Here's how the part is built. I have some questions about the finished solid (model axes, mm). A direction names the side the tool comes from. Round coordinates to 2 decimals unless told otherwise and drop trailing zeros. Loops run counter-clockwise (first coordinate to the right, second up) from the corner with the lowest first, then second, coordinate; pieces in that order, holes last. Notation, with made-up numbers: M 51.5,78 L 73.5,78 A14 cw 73.5,105 Z; hole C 33.5,-7.75 d8. An arc over 180 degrees is marked long. Put each result on its own line as item: value. Start each with the question number.
```python
from build123d import *

# Parameters (mm, degrees)
F0_R      = 5.1
F1_DEPTH  = 35
F2_W      = 22
F2_H      = 9.65
F3_DEPTH  = 35
F4_DEPTH  = 5
F5_DEPTH  = 2.5
F6_R      = 1.9
F7_DEPTH  = 20
F6_R_2    = 2.65
F8_DEPTH  = 2
F10_DEPTH = 35
F11_COUNT = 3


with BuildPart() as f1:
    # F0 (on Top) → F1 (new body)
    with BuildSketch(Plane.XY):
        with BuildLine():
            Line((48.3891499996, -27.9374887781), (0, 0))
            Line((0, 0), (-48.3891499996, -27.9374887781))
            ThreePointArc((-48.3891499996, -27.9374887781), (-37.0005953155, -59.5433683199), (-37.3249107961, -93.1369036932))
            ThreePointArc((-37.3249107961, -93.1369036932), (-26.5643472762, -85.0438685233), (-17.5, -95))
            ThreePointArc((-17.5, -95), (-20.4289321881, -102.0710678119), (-27.5, -105))
            Line((-27.5, -105), (27.5, -105))
            ThreePointArc((27.5, -105), (19.7983455327, -88.6215583043), (37.3249107961, -93.1369036932))
            ThreePointArc((37.3249107961, -93.1369036932), (37.0005953155, -59.5433683199), (48.3891499996, -27.9374887781))
        make_face()
        with BuildLine():
            ThreePointArc((37.5, -95), (37.4561314767, -94.0643472762), (37.3249107961, -93.1369036932))
            ThreePointArc((37.3249107961, -93.1369036932), (19.7983455327, -88.6215583043), (27.5, -105))
            ThreePointArc((27.5, -105), (34.5710678119, -102.0710678119), (37.5, -95))
        make_face()
        with Locations((27.5, -95)):
            Circle(F0_R, mode=Mode.SUBTRACT)
        with BuildLine():
            ThreePointArc((-17.5, -95), (-26.5643472762, -85.0438685233), (-37.3249107961, -93.1369036932))
            ThreePointArc((-37.3249107961, -93.1369036932), (-35.2016544673, -101.3784416957), (-27.5, -105))
            ThreePointArc((-27.5, -105), (-20.4289321881, -102.0710678119), (-17.5, -95))
        make_face()
        with Locations((-27.5, -95)):
            Circle(F0_R, mode=Mode.SUBTRACT)
    extrude(amount=-F1_DEPTH)

    # F2 (on face) → F3 (cut, through all)
    with BuildSketch(Plane.XY):
        with Locations((0, -95.005)):
            Rectangle(F2_W, F2_H)
    extrude(amount=-F3_DEPTH, mode=Mode.SUBTRACT)

    # F2 (on face) → F4 (join)
    with BuildSketch(Plane.XY):
        with Locations((0, -95.005)):
            Rectangle(F2_W, F2_H)
    extrude(amount=-F4_DEPTH)

    # F0 (on Top) → F5 (join)
    with BuildSketch(Plane.XY):
        with Locations((27.5, -95)):
            Circle(F0_R)
        with Locations((-27.5, -95)):
            Circle(F0_R)
    extrude(amount=-F5_DEPTH)

    # F6 (on face) → F7 (cut)
    with BuildSketch(Plane.XZ.offset(105)):
        with Locations((0, -20)):
            Circle(F6_R)
    extrude(amount=-F7_DEPTH, mode=Mode.SUBTRACT)

    # F6 (on face) → F8 (cut)
    with BuildSketch(Plane.XZ.offset(105)):
        with Locations((0, -20)):
            Circle(F6_R_2)
        with Locations((0, -20)):
            Circle(F6_R, mode=Mode.SUBTRACT)
    extrude(amount=-F8_DEPTH, mode=Mode.SUBTRACT)

    # F9 (on face) → F10 (cut, through all)
    with BuildSketch(Plane(origin=(0, 0, -35), x_dir=(1, 0, 0), z_dir=(0, 0, -1))):
        Polygon((20.0250012255, 95.005), (20.0250012255, 99.83), (13.3750012255, 99.83), (13.3750012255, 95.005), (13.3750012255, 79.43), (20.0250012255, 79.43), align=None)
    extrude(amount=-F10_DEPTH, mode=Mode.SUBTRACT)

    # F11: F1 ×3 about axis
    f11_axis = Axis((0, 0, 0), (0, 0, 1))


with BuildPart() as f1_1:
    add(f1.part)
    for i in range(1, F11_COUNT):
        add(f1.part.rotate(f11_axis, i * 360 / F11_COUNT))


solid = f1_1.part
```
1) Suppose I cut it at A-A (y = -47). Write out the boundary of the cut face in (x, z), plus the area to 3 significant figures.
2) I'm going to push flat-ended pins straight in: P1, Ø1, axis at x = 70, z = -22, coming from the +Y side; P2, Ø5.5, axis at x = 17.5, z = -23, coming from the +Y side; P3, Ø6, axis at x = -68.52, y = 71.32, coming from the -Z side. Where does each tip first touch, or does it pass through?
3) Suppose I cut it at B-B (z = -25). State how many separate pieces and enclosed holes the cut face has, plus the area to 3 significant figures.
4) If I drill on probe 1 along Z at (x, y) = (0, -87.25); probe 2 along Y at (x, z) = (-84.5, -27.5); probe 3 along X at (y, z) = (36, -18.5), over which ranges is the centre line in solid material (lowest first)? Write a range as from..to.
5) On a 3-axis mill with a long thin cutter (end or side, diameter ignored), from which of +Z, -Z, +X, -X, +Y, -Y can I reach the whole of each face in a straight line? I mean faces 1 (the face through (13.375, -90, -18)), 2 (the face through (-90.065, 50.002, -21.141)), 3 (the face through (27, -95, -2.5)). Say none if no direction works.
6) If we mould it in two halves opening along Z, with no side actions, what happens to faces 4 (the face through (10, -4, -35)), 5 (the face through (-90.791, 50.773, -17.766)), 6 (the face through (-0.34, -104.01, -17.37)), 7 (the face through (20.025, -89, -18))? For each: pulls with the +Z half, pulls with the -Z half, needs draft (parallel to the pull), parting line crosses it, or undercut.
Results are:
1. outline: M -40.02,-35 L 40.02,-35 L 40.02,0 L -40.02,0 Z
1. area: 2,800 mm²
2. P1: y = 81.27
2. P2: y = 58.06
2. P3: z = -2.5
3. separate pieces: 1
3. enclosed holes: 12
3. area: 20,200 mm²
4. probe 1: -35..-21.9, -18.1..0
4. probe 2: 7.59..25.66, 33.34..36.08, 53.3..63.64
4. probe 3: -100.46..-94.49, -89.1..-84.35, -83.35..83.35, 84.35..100.46
5. face 1: +Z, -Z
5. face 2: none
5. face 3: -Z
6. face 4: pulls with the -Z half
6. face 5: undercut
6. face 6: undercut
6. face 7: needs draft
